Can you work these out from the drawing? Everything is in mm from the part's minimum corner. A direction names the side the tool comes from. Coordinates: 2 decimals unless noted, no trailing zeros. Loops run counter-clockwise (first coordinate to the right, second up) from the corner with the lowest first, then second, coordinate; pieces in that order, holes last. Notation, with made-up numbers: (-6.5, 44) - (12.5, 44) arc R24 cw to (12.5, 59) - close; hole circle Ø10 at (-32.75, 14.25). An arc over 180 degrees is marked (long way). Use CSV: the item, a comma, the result in double quotes.
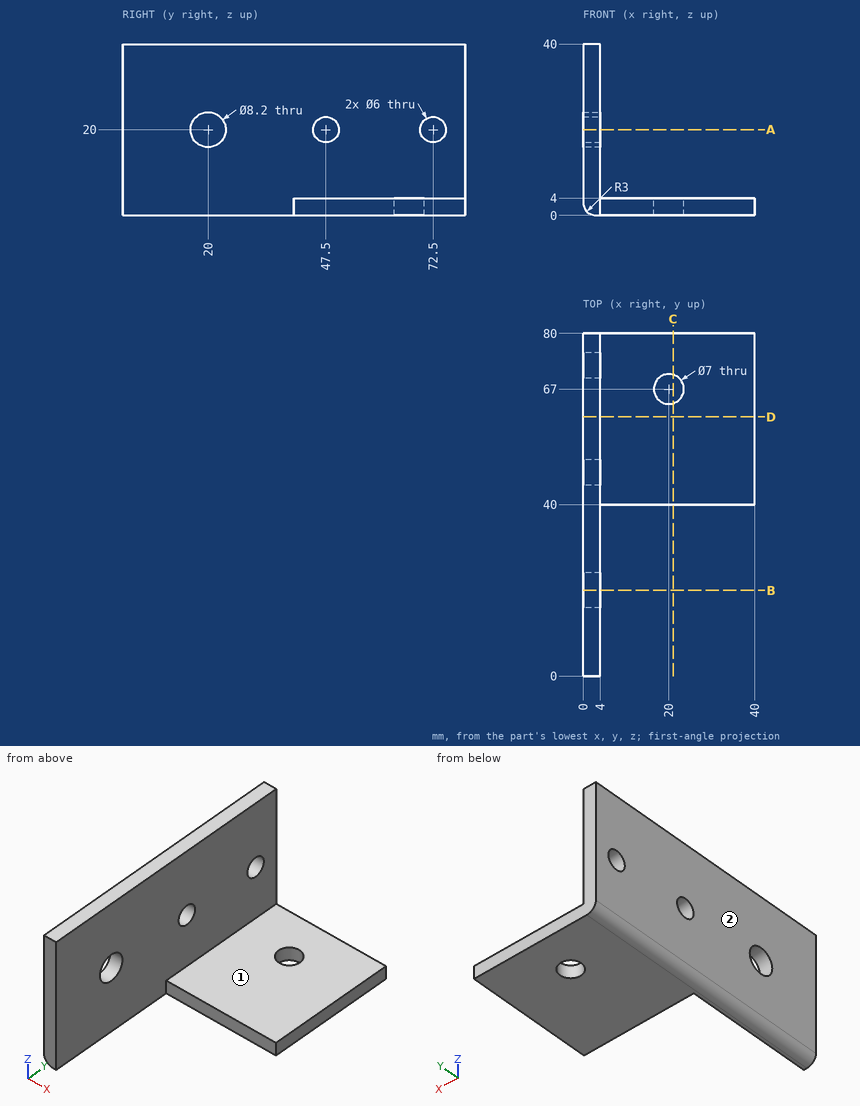
(1) Suppose I cut it at D-D (y = 60.5). Write out the boundary of the cut face in (x, z), plus the area to 3 significant figures.
Computed:
outline,"(0, 3) arc R3 ccw to (3, 0) - (40, 0) - (40, 4) - (4, 4) - (4, 40) - (0, 40) - close"
area,"302 mm²"
(2) Suppose I cut it at A-A (z = 20). Write out the boundary of the cut face in (x, y), plus the area to 3 significant figures.
Computed:
outline,"(0, 0) - (4, 0) - (4, 15.9) - (0, 15.9) - close; (0, 24.1) - (4, 24.1) - (4, 44.5) - (0, 44.5) - close; (0, 50.5) - (4, 50.5) - (4, 69.5) - (0, 69.5) - close; (0, 75.5) - (4, 75.5) - (4, 80) - (0, 80) - close"
area,"239 mm²"
(3) Please list where these lines run through material, in increasing order: line 1 (Y direction, x = 1, z = 20); line 2 (Z direction, x = 12.5, y = 75).
Computed:
line 1,"y = 0 to 15.9, 24.1 to 44.5, 50.5 to 69.5, 75.5 to 80"
line 2,"z = 0 to 4"
(4) Will these pins go through, and if not, where does the flat tip stop? pin 1 (9.5 mm diameter, centred on y = 47.5, z = 20, fed in from +X); pin 2 (11 mm diameter, centred on x = 24, y = 67, fed in from +Z); pin 3 (5 mm diameter, centred on y = 20, z = 20, fed in from +X); pin 4 (4.5 mm diameter, centred on x = 28, z = 1, fed in from -Y).
Computed:
pin 1,"stops at x = 4"
pin 2,"stops at z = 4"
pin 3,"passes through"
pin 4,"stops at y = 40"
(5) Which directions (+Z, -Z, +X, -X, +Y, -Y) give clear straight access to the entire face, cutting with the end or side of a thin tool? Please do the marked faces 1 and 2.
Computed:
face 1,"+Z, +X, +Y, -Y"
face 2,"+Z, -Z, -X, +Y, -Y"
(6) Suppose I cut it at C-C (x = 21). Write out the boundary of the cut face in (y, z), plus the area to 3 significant figures.
Computed:
outline,"(40, 0) - (63.65, 0) - (63.65, 4) - (40, 4) - close; (70.35, 0) - (80, 0) - (80, 4) - (70.35, 4) - close"
area,"133 mm²"
(7) Suppose I cut it at B-B (y = 20). Write out the boundary of the cut face in (x, z), plus the area to 3 significant figures.
Computed:
outline,"(0, 3) arc R3 ccw to (3, 0) - (4, 0) - (4, 15.9) - (0, 15.9) - close; (0, 24.1) - (4, 24.1) - (4, 40) - (0, 40) - close"
area,"125 mm²"
